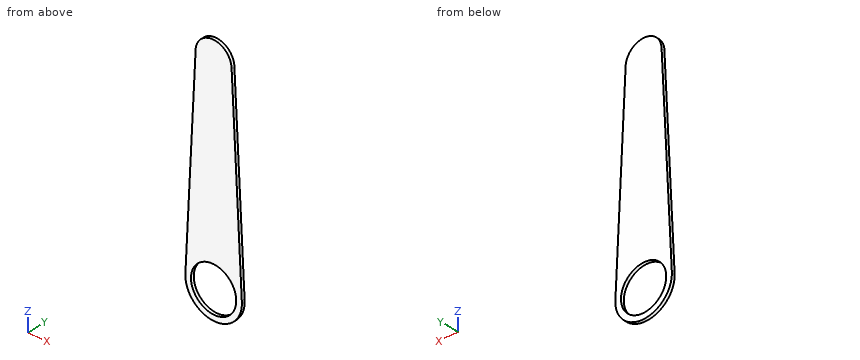
```python
from build123d import *

# Parameters (mm, degrees)
SKETCH1_R           = 17.5
BOSS_EXTRUDE1_DEPTH = 3
SKETCH2_R           = 22
CUT_EXTRUDE1_DEPTH  = 220.25213796


with BuildPart() as part:
    # Sketch1 → Boss-Extrude1 (new body)
    with BuildSketch(Plane(origin=(0, 0, 0), x_dir=(1, 0, 0), z_dir=(0, 1, 0))):
        with BuildLine():
            ThreePointArc((27.5, 0), (0, 27.5), (-27.5, 0))
            Line((-27.5, 0), (-27.362842893, -2.743142145))
            ThreePointArc((-27.362842893, -2.743142145), (0, -27.5), (27.362842893, -2.743142145))
            Line((27.362842893, -2.743142145), (27.5, 0))
        make_face()
        with BuildLine():
            ThreePointArc((27.362842893, -2.743142145), (0, -27.5), (-27.362842893, -2.743142145))
            Line((-27.362842893, -2.743142145), (-17.5, -200))
            ThreePointArc((-17.5, -200), (0, -182.5), (17.5, -200))
            Line((17.5, -200), (27.362842893, -2.743142145))
        make_face()
        with Locations((0, -200)):
            Circle(SKETCH1_R)
    extrude(amount=BOSS_EXTRUDE1_DEPTH)

    # Sketch2 → Cut-Extrude1 (cut, through all)
    with BuildSketch(Plane(origin=(0, 3, 0), x_dir=(1, 0, 0), z_dir=(0, 1, 0))):
        with Locations(Location((0, 0, 0), (0, 0, 270))):
            Circle(SKETCH2_R)
    extrude(amount=-CUT_EXTRUDE1_DEPTH, mode=Mode.SUBTRACT)


solid = part.part
```
CAD build for the part. Positions are in the model's coordinates, mm. Coordinates: 2 decimals unless noted, no trailing zeros. Write each loop counter-clockwise with the first axis right and the second up, starting at its lowest first coordinate (ties: lowest second). Pieces come first, ordered by that corner, then holes.
(1) Cut at B-B, the plane z = -5. List the corners of the cut face in (x, y).
(2) Cut at A-A, the plane x = 0. List the corners of the cut face in (y, z).
(3) Drill centre lines: probe 1 along X at (y, z) = (2.3, 0); probe 2 along Z at (x, y) = (-11, 0.9); probe 3 along X at (y, z) = (1, -16). Where is each one in solid material? Low to high.
(4) Cut at C-C, the plane y = 0.6. List the corners of the cut face in (x, z), and give its area (3 significant figures).
(5) Cut at D-D, the plane z = 56. List the corners of the cut face in (x, y).
Geometry says:
1. outline: (-27.04, 0) - (-21.42, 0) - (-21.42, 3) - (-27.04, 3) - close; (21.42, 0) - (27.04, 0) - (27.04, 3) - (21.42, 3) - close
2. outline: (0, -27.5) - (3, -27.5) - (3, -22) - (0, -22) - close; (0, 22) - (3, 22) - (3, 217.5) - (0, 217.5) - close
3. probe 1: x = -27.5 to -22, 22 to 27.5
3. probe 2: z = -25.2 to -19.05, 19.05 to 213.61
3. probe 3: x = -22.37 to -15.1, 15.1 to 22.37
4. outline: (-27.5, 0) arc R27.5 ccw to (27.5, 0) - (17.5, 200) arc R17.5 ccw to (-17.5, 200) - close; hole circle Ø44 at (0, 0)
4. area: 9,150 mm2
5. outline: (-24.7, 0) - (24.7, 0) - (24.7, 3) - (-24.7, 3) - close
